Source: CAD feature listing. Evaluate the final solid. Frame: model axes, mm. Face numbers are marked on the shaded views. A direction names the side the tool comes from. Coordinates: 2 decimals unless noted, no trailing zeros. Order: outer loops, then holes, each group sorted by start corner. A loop starts at its lowest first (then second) coordinate and runs counter-clockwise, first axis right, second up.
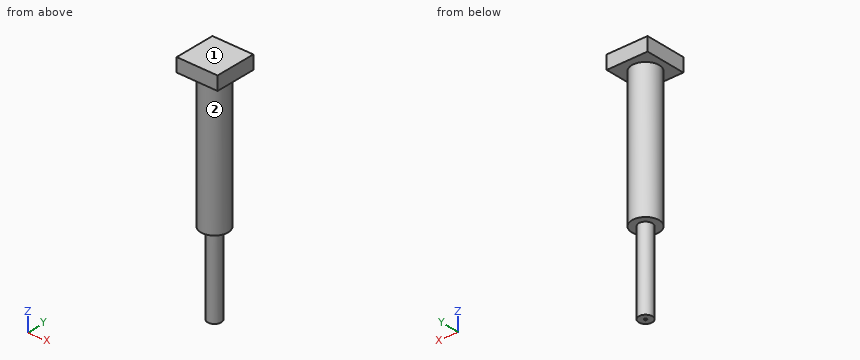
```python
from build123d import *

# Parameters (mm, degrees)
F0_W     = 7.62
F0_H     = 7.62
F1_DEPTH = 2.54
F2_R     = 1.27
F3_DEPTH = 40.64
F4_R     = 0.254
F5_DEPTH = 2.54
F2_R_2   = 2.54
F6_DEPTH = 25.4


with BuildPart() as f1:
    # F0 (on Top) → F1 (new body)
    with BuildSketch(Plane.XY):
        with Locations((-38.795546, -21.835937)):
            Rectangle(F0_W, F0_H)
    extrude(amount=F1_DEPTH)

    # F2 (on face) → F3 (join)
    with BuildSketch(Plane(origin=(0, 0, 0), x_dir=(1, 0, 0), z_dir=(0, 0, -1))):
        with Locations((-38.854431, 21.888208)):
            Circle(F2_R)
    extrude(amount=F3_DEPTH)

    # F4 (on face) → F5 (cut)
    with BuildSketch(Plane(origin=(0, 0, -40.64), x_dir=(1, 0, 0), z_dir=(0, 0, -1))):
        with Locations((-38.854431, 21.888208)):
            Circle(F4_R)
    extrude(amount=-F5_DEPTH, mode=Mode.SUBTRACT)

    # F2 (on face) → F6 (join)
    with BuildSketch(Plane(origin=(0, 0, 0), x_dir=(1, 0, 0), z_dir=(0, 0, -1))):
        with Locations((-38.854431, 21.888208)):
            Circle(F2_R_2)
        with Locations((-38.854431, 21.888208)):
            Circle(F2_R, mode=Mode.SUBTRACT)
    extrude(amount=F6_DEPTH)


solid = f1.part
```
1. Section query D-D, the plane x = -40.75. Output: boundary loops of the cut face in (y, z).
2. Section query A-A, the plane x = -36.75. Output: boundary loops of the cut face in (y, z), plus the area to 3 significant figures.
3. Section query C-C, the plane z = -30.5. Output: boundary loops of the cut face in (x, y).
4. Section query B-B, the plane y = -22.5. Output: boundary loops of the cut face in (x, z).
5. Material intervals for line 1 along Z through (x, y) = (-42, -24.25); line 2 along Z through (x, y) = (-40.75, -20.5); line 3 along Y through (x, z) = (-38, -1.5), sorted ascending.
6. Access query for the marked faces 1 and 2. Directions: +Z, -Z, +X, -X, +Y, -Y. A direction counts if a zero-diameter tool reaches every point of the face in a straight line with its end or side. Return the directions, or none.
7. Contact query for flat-ended pins moving along their axis: P1, Ø1, axis at x = -36.5, z = -21.5, coming from the +Y side; P2, Ø3, axis at x = -36.5, z = -13, coming from the +Y side; P3, Ø2, axis at y = -23.5, z = -20.5, coming from the -X side. Output: stop coordinate, or through.
Answer key:
1. outline: (-25.65, 0) - (-23.58, 0) - (-23.58, -25.4) - (-20.2, -25.4) - (-20.2, 0) - (-18.03, 0) - (-18.03, 2.54) - (-25.65, 2.54) - close
2. outline: (-25.65, 0) - (-23.31, 0) - (-23.31, -25.4) - (-20.47, -25.4) - (-20.47, 0) - (-18.03, 0) - (-18.03, 2.54) - (-25.65, 2.54) - close
2. area: 91.6 mm2
3. outline: circle Ø2.54 at (-38.85, -21.89)
4. outline: (-42.61, 0) - (-41.32, 0) - (-41.32, -25.4) - (-39.97, -25.4) - (-39.97, -40.64) - (-37.74, -40.64) - (-37.74, -25.4) - (-36.39, -25.4) - (-36.39, 0) - (-34.99, 0) - (-34.99, 2.54) - (-42.61, 2.54) - close
5. line 1: z = 0 to 2.54
5. line 2: z = -25.4 to 2.54
5. line 3: y = -24.28 to -19.5
6. face 1: +Z, +X, -X, +Y, -Y
6. face 2: -Z
7. P1: stops at y = -20.15
7. P2: stops at y = -19.5
7. P3: stops at x = -41.32
